Input: part model. Units: mm. Frame: model coordinates. A direction names the side the tool comes from. Give positions to 0.01 mm unless a question says otherwise; leave off trailing zeros. Loops run counter-clockwise (first coordinate to the right, second up) from the corner with the lowest first, then second, coordinate; pieces in that order, holes last. Notation, with made-up numbers: M 40,19 L 99,19 A17 cw 99,42 Z; hole C 58,71 d5. An arc over 180 degrees is marked long. Use a Markdown table: item, result. Add a question column.
from build123d import *

# Parameters (mm, degrees)
SKETCH1_R           = 3
SKETCH1_R_2         = 1.5
BOSS_EXTRUDE1_DEPTH = 6


with BuildPart() as part:
    # Sketch1 → Boss-Extrude1 (new body)
    with BuildSketch(Plane(origin=(0, 0, 0), x_dir=(1, 0, 0), z_dir=(0, 1, 0))):
        Polygon((-72, 72), (-72, 28), (-66, 28), (-66, 4.5), (-62, 4.5), (-62, 6.5), (-59, 6.5), (-59, 4.5), (-56, 4.5), (-56, 1.5), (-59, 1.5), (-59, -0.5), (-62, -0.5), (-62, 1.5), (-66, 1.5), (-66, -22), (-72, -22), (-72, -72), (-22, -72), (-22, -66), (1.5, -66), (1.5, -62), (-0.5, -62), (-0.5, -59), (1.5, -59), (1.5, -56), (4.5, -56), (4.5, -59), (6.5, -59), (6.5, -62), (4.5, -62), (4.5, -66), (28, -66), (28, -72), (72, -72), (72, -22), (78, -22), (78, 28), (72, 28), (72, 72), (28, 72), (28, 78), (-22, 78), (-22, 72), align=None)
        with Locations(Location((3, 3, 0), (0, 0, 270))):
            Circle(SKETCH1_R, mode=Mode.SUBTRACT)
        with Locations(Location((25.5, 3, 0), (0, 0, 270))):
            Circle(SKETCH1_R, mode=Mode.SUBTRACT)
        with Locations(Location((3, 75, 0), (0, 0, 270))):
            Circle(SKETCH1_R_2, mode=Mode.SUBTRACT)
        with Locations(Location((75, 3, 0), (0, 0, 270))):
            Circle(SKETCH1_R_2, mode=Mode.SUBTRACT)
    extrude(amount=BOSS_EXTRUDE1_DEPTH)


solid = part.part
1) Ray query, line 1 (X direction, y = 2, z = -3); line 2 (X direction, y = 2.85, z = 65.5); line 3 (X direction, y = 4.8, z = -3.5). Return the intervals inside material, ascending. Write a range as [from, to].
2) Section query A-A, the plane x = 25.5. Return the cut outline in (y, z), and give its area (3 significant figures).
3) Pull-direction query (X, two-part tool) for faces 1 (the cylindrical face through (27.53, 2.96, -5.21)), 2 (the flat face through (-66, 3, -16)), 3 (the cylindrical face through (5.03, 2.96, -5.21)), 4 (the flat face through (-69, 3, -28)); classes: pulls with the +X half, pulls with the -X half, needs draft (parallel to the pull), parting line crosses it, or undercut.
4) Section query D-D, the plane x = -42. Return the cut outline in (y, z), and give its area (3 significant figures).
5) Contact query for flat-ended pins moving along their axis: P1, Ø1.5, axis at x = -57.5, y = 4.5, coming from the -Z side; P2, Ø0.6, axis at y = 2, z = -5, coming from the -X side; P3, Ø0.9, axis at y = 2.5, z = -3.5, coming from the -X side. Output: stop coordinate, or through.
6) Reachability of faces 5 (the flat face through (-64, 3, -4.5)), 6 (the flat face through (-22, 3, -75)), 7 (the flat face through (72, 3, -50)), 8 (the flat face through (-22, 3, 69)) from +Z, -Z, +X, -X, +Y, -Y: full face, straight path, thin tool, end or side. Return the list, or none.
7) Section query C-C, the plane z = 36.5. Return the cut outline in (x, y).
8) Section query B-B, the plane y = 1.5. State how many separate pieces and enclosed holes the cut face has, and give its area (3 significant figures).
Entries:
| question | item | result |
|---|---|---|
| 1 | line 1 | x = [-56, 0], [6, 22.5], [28.5, 73.5], [76.5, 78] |
| 1 | line 2 | x = [-72, 1.5], [4.5, 72] |
| 1 | line 3 | x = [-56, 0.04], [5.96, 22.54], [28.46, 73.59], [76.41, 78] |
| 2 | outline | M 0,-78 L 6,-78 L 6,-6 L 0,-6 Z; M 0,0 L 6,0 L 6,66 L 0,66 Z |
| 2 | area | 828 mm² |
| 3 | face 1 | undercut |
| 3 | face 2 | pulls with the -X half |
| 3 | face 3 | undercut |
| 3 | face 4 | needs draft |
| 4 | outline | M 0,-72 L 6,-72 L 6,72 L 0,72 Z |
| 4 | area | 864 mm² |
| 5 | P1 | stops at z = -72 |
| 5 | P2 | stops at x = -66 |
| 5 | P3 | stops at x = -56 |
| 6 | face 5 | -X, +Y, -Y |
| 6 | face 6 | -Z, -X, +Y, -Y |
| 6 | face 7 | -Z, +X, +Y, -Y |
| 6 | face 8 | +Z, +Y, -Y |
| 7 | outline | M -72,0 L 72,0 L 72,6 L -72,6 Z |
| 8 | separate pieces | 1 |
| 8 | enclosed holes | 4 |
| 8 | area | 20,600 mm² |
